```python
from build123d import *

# Parameters (mm, degrees)
SKETCH1_W                                           = 100
SKETCH1_H                                           = 110
BOSS_EXTRUDE1_DEPTH                                 = 8
CBORE_FOR_M3_HEX_SOCKET_HEAD_CAP_SCREW1_D           = 3.4
CBORE_FOR_M3_HEX_SOCKET_HEAD_CAP_SCREW1_DEPTH       = 8
CBORE_FOR_M3_HEX_SOCKET_HEAD_CAP_SCREW1_CBORE_D     = 6.5
CBORE_FOR_M3_HEX_SOCKET_HEAD_CAP_SCREW1_CBORE_DEPTH = 3.4
CBORE_FOR_M3_HEX_SOCKET_HEAD_CAP_SCREW1_TIP         = 1.021463052
F_30_0_30_DIAMETER_HOLE1_D                          = 30
F_30_0_30_DIAMETER_HOLE1_DEPTH                      = 10
F_30_0_30_DIAMETER_HOLE1_TIP                        = 9.012909285
SKETCH7_R                                           = 35.3
CUT_EXTRUDE1_DEPTH                                  = 4.5
M4_CLEARANCE_HOLE1_D                                = 4.5
CUT_EXTRUDE2_DEPTH                                  = 6
FILLET1_R                                           = 4


with BuildPart() as part:
    # Sketch1 → Boss-Extrude1 (new body)
    with BuildSketch(Plane(origin=(0, 0, 0), x_dir=(1, 0, 0), z_dir=(0, 1, 0))):
        with Locations((50, 55)):
            Rectangle(SKETCH1_W, SKETCH1_H)
    extrude(amount=BOSS_EXTRUDE1_DEPTH)

    # CBORE for M3 Hex Socket Head Cap Screw1
    with Locations(Plane(origin=(0, 8, 0), x_dir=(1, 0, 0), z_dir=(0, 1, 0))):
        with Locations((96, 105), (6.2, 105), (6.2, 80), (6.2, 55), (6.2, 30), (6.2, 5), (96, 55), (96, 30), (96, 5), (96, 80)):
            CounterBoreHole(CBORE_FOR_M3_HEX_SOCKET_HEAD_CAP_SCREW1_D / 2, CBORE_FOR_M3_HEX_SOCKET_HEAD_CAP_SCREW1_CBORE_D / 2, CBORE_FOR_M3_HEX_SOCKET_HEAD_CAP_SCREW1_CBORE_DEPTH, depth=CBORE_FOR_M3_HEX_SOCKET_HEAD_CAP_SCREW1_DEPTH)
            with Locations((0, 0, -(CBORE_FOR_M3_HEX_SOCKET_HEAD_CAP_SCREW1_DEPTH + CBORE_FOR_M3_HEX_SOCKET_HEAD_CAP_SCREW1_TIP / 2))):  # 118° drill point
                Cone(0, CBORE_FOR_M3_HEX_SOCKET_HEAD_CAP_SCREW1_D / 2, CBORE_FOR_M3_HEX_SOCKET_HEAD_CAP_SCREW1_TIP, mode=Mode.SUBTRACT)

    # Ø30.0 (30) Diameter Hole1
    with Locations(Plane(origin=(0, 8, 0), x_dir=(1, 0, 0), z_dir=(0, 1, 0))):
        with Locations((50, 55)):
            Hole(F_30_0_30_DIAMETER_HOLE1_D / 2, depth=F_30_0_30_DIAMETER_HOLE1_DEPTH)
            with Locations((0, 0, -(F_30_0_30_DIAMETER_HOLE1_DEPTH + F_30_0_30_DIAMETER_HOLE1_TIP / 2))):  # 118° drill point
                Cone(0, F_30_0_30_DIAMETER_HOLE1_D / 2, F_30_0_30_DIAMETER_HOLE1_TIP, mode=Mode.SUBTRACT)

    # Sketch7 → Cut-Extrude1 (cut)
    with BuildSketch(Plane(origin=(0, 8, 0), x_dir=(1, 0, 0), z_dir=(0, 1, 0))):
        with Locations(Location((50, 55, 0), (0, 0, 270))):
            Circle(SKETCH7_R)
    extrude(amount=-CUT_EXTRUDE1_DEPTH, mode=Mode.SUBTRACT)

    # M4 Clearance Hole1 (through all)
    with Locations(Plane(origin=(0, 0, 0), x_dir=(-1, 0, 0), z_dir=(0, -1, 0))):
        with Locations((-64.142135624, 69.142135624), (-50, 75), (-35.857864376, 69.142135624), (-30, 55), (-35.857864376, 40.857864376), (-50, 35), (-64.142135624, 40.857864376), (-70, 55)):
            Hole(M4_CLEARANCE_HOLE1_D / 2)

    # Sketch12 → Cut-Extrude2 (cut)
    with BuildSketch(Plane(origin=(0, 8, 0), x_dir=(1, 0, 0), z_dir=(0, 1, 0))):
        with BuildLine():
            Line((87, 105), (13, 105))
            Line((13, 105), (13, 70.971537183))
            ThreePointArc((13, 70.971537183), (50, 95.3), (87, 70.971537183))
            Line((87, 70.971537183), (87, 105))
        make_face()
        with BuildLine():
            ThreePointArc((87, 39.028462817), (50, 14.7), (13, 39.028462817))
            Line((13, 39.028462817), (13, 5))
            Line((13, 5), (87, 5))
            Line((87, 5), (87, 39.028462817))
        make_face()
    extrude(amount=-CUT_EXTRUDE2_DEPTH, mode=Mode.SUBTRACT)

    # Fillet1
    fillet1_edges = [part.edges().sort_by_distance(p)[0] for p in [
        (87, 5, -70.971537183),
        (13, 5, -70.971537183),
        (13, 5, -105),
        (87, 5, -105),
        (13, 5, -39.028462817),
        (87, 5, -39.028462817),
        (87, 5, -5),
        (13, 5, -5),
    ]]
    fillet(fillet1_edges, radius=FILLET1_R)


solid = part.part
```
Input: part model. Units: mm. Frame: model coordinates. A direction names the side the tool comes from. Give positions to 0.01 mm unless a question says otherwise; leave off trailing zeros. Order: outer loops, then holes, each group sorted by start corner. A loop starts at its lowest first (then second) coordinate and runs counter-clockwise, first axis right, second up. Notation, with made-up numbers: (-14.5, -20) - (-2.5, -20) arc R11 cw to (-2.5, 1) - close; hole circle Ø8 at (6.25, 68.5). An arc over 180 degrees is marked (long way). Use a Markdown table: item, result.
(1) Pin query (flat end, axial travel): pin 1 (4.5 mm diameter, centred on x = 96, z = -105, fed in from +Y); pin 2 (2 mm diameter, centred on x = 66.5, z = -15, fed in from +Y); pin 3 (3 mm diameter, centred on x = 36.5, z = -44, fed in from +Y). Return the tip coordinate at first contact, or that it passes through.
Computed values:
| item | result |
|---|---|
| pin 1 | stops at y = 4.6 |
| pin 2 | stops at y = 2 |
| pin 3 | stops at y = 3.5 |
(2) Line query: line 1 (Z direction, x = 6.2, y = 7); line 2 (Z direction, x = 83, y = 2.75); line 3 (Z direction, x = 50, y = 0.9). Output: solid intervals per line, ascending. Write a range as from..to.
Computed values:
| item | result |
|---|---|
| line 1 | z = -110..-108.25, -101.75..-83.25, -76.75..-58.25, -51.75..-33.25, -26.75..-8.25, -1.75..0 |
| line 2 | z = -110..-105, -80.55..-29.45, -5..0 |
| line 3 | z = -110..-77.25, -72.75..-70, -40..-37.25, -32.75..0 |
(3) Access query for faces 1 (the cylindrical face through (97.35, 2.27, -103.97)), 2 (the cylindrical face through (84.365, 4.958, -29.205)). Directions: +Z, -Z, +X, -X, +Y, -Y. A direction counts if a zero-diameter tool reaches every point of the face in a straight line with its end or side. Return the directions, or none.
Computed values:
| item | result |
|---|---|
| face 1 | +Y, -Y |
| face 2 | +Y |
(4) Draft query along Z for faces 3 (the cylindrical face through (71.21, 1.774, -56.897)), 4 (the flat face through (60.4, 0, -43.5)). Return one class per face: released by +Z, released by -Z, zero draft, split by the parting line, or undercut.
Computed values:
| item | result |
|---|---|
| face 3 | undercut |
| face 4 | zero draft |
(5) Section query A-A (y = 6.75). State how many separate pieces and enclosed holes the cut face has, then the cut area to 3 significant figures.
Computed values:
| item | result |
|---|---|
| separate pieces | 1 |
| enclosed holes | 13 |
| area | 4,440 mm2 |
(6) Section query C-C (z = -35). Output: boundary loops of the cut face in (x, y), then the cut area to 3 significant figures.
Computed values:
| item | result |
|---|---|
| outline | (0, 0) - (47.75, 0) - (47.75, 3.5) - (20.91, 3.5) - (20.91, 8) - (0, 8) - close; (52.25, 0) - (100, 0) - (100, 8) - (79.09, 8) - (79.09, 3.5) - (52.25, 3.5) - close |
| area | 522 mm2 |
(7) Section query B-B (x = 45). Output: boundary loops of the cut face in (y, z).
Computed values:
| item | result |
|---|---|
| outline | (0, -110) - (8, -110) - (8, -105) - (2, -105) - (2, -94.99) - (8, -94.99) - (8, -89.94) - (3.5, -89.94) - (3.5, -69.14) - (0, -69.14) - close; (0, -40.86) - (3.5, -40.86) - (3.5, -20.06) - (8, -20.06) - (8, -15.01) - (2, -15.01) - (2, -5) - (8, -5) - (8, 0) - (0, 0) - close |
